Answer from the drawing. Dimensions are ordinates in mm from the lowest x, y and z of the part. A direction names the side the tool comes from. Round coordinates to 2 decimals unless told otherwise and drop trailing zeros. Loops run counter-clockwise (first coordinate to the right, second up) from the corner with the lowest first, then second, coordinate; pieces in that order, holes last. Notation, with made-up numbers: (33.25, -7.75) - (46.25, -7.75) arc R20 cw to (46.25, 16.25) - close; hole circle Ø10 at (-30.75, -10). An arc over 180 degrees is marked (long way). Use CSV: the item, a comma, the result in double quotes. Start each with the question number.
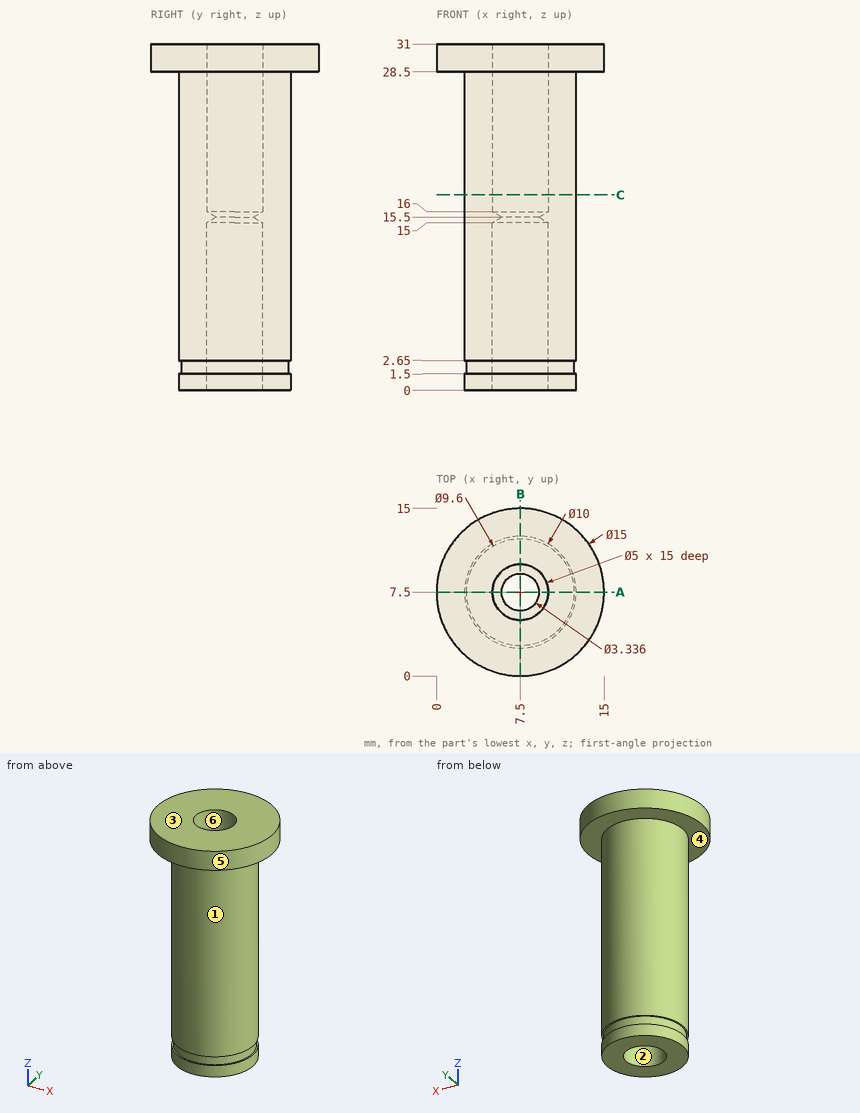
Item 1: The mould has two halves that part along Y. Classify the marked faces 1, 2 and 3: pulls with the +Y half, pulls with the -Y half, needs draft (parallel to the pull), parting line crosses it, or undercut.
Item 2: Find the intervals of material crossed by probe 1 along X at (y, z) = (7.5, 11); probe 2 along Z at (x, y) = (12, 3.25), in increasing order. Write a range as [from, to].
Item 3: Which of the six approach directions +Z, -Z, +X, -X, +Y, -Y give full straight-line access (tool end or side, diameter ignored) to the marked faces 4, 5 and 6?
Item 4: A cutting plane is placed at C-C (z = 17.5). Determine the outline of the cut face in (x, y), plus the area to 3 significant figures.
Item 5: A cutting plane is placed at A-A (y = 7.5). Determine the outline of the cut face in (x, z).
Item 6: Each of these flat-tipped pins is pushed along its axis until it touches: pin 1 Ø4 at (x, y) = (7.5, 7.5) entering from -Z; pin 2 Ø8 at (x, z) = (11.5, 22.5) entering from -Y; pin 3 Ø8 at (x, y) = (7.5, 7.5) entering from -Z; pin 4 Ø8 at (x, z) = (12, 6.5) entering from +Y (3 decimals). Where does it stop, or does it pass through?
Result sheet:
1,face 1,"parting line crosses it"
1,face 2,"undercut"
1,face 3,"needs draft"
2,probe 1,"[2.5, 5], [10, 12.5]"
2,probe 2,"[28.5, 31]"
3,face 4,"-Z"
3,face 5,"+Z, -Z"
3,face 6,"+Z"
4,outline,"circle Ø10 at (7.5, 7.5); hole circle Ø5 at (7.5, 7.5)"
4,area,"58.9 mm^2"
5,outline,"(0, 28.5) - (2.5, 28.5) - (2.5, 2.65) - (2.7, 2.65) - (2.7, 1.5) - (2.5, 1.5) - (2.5, 0) - (5, 0) - (5, 15) - (5.83, 15.5) - (5, 16) - (5, 31) - (0, 31) - close; (9.17, 15.5) - (10, 15) - (10, 0) - (12.5, 0) - (12.5, 1.5) - (12.3, 1.5) - (12.3, 2.65) - (12.5, 2.65) - (12.5, 28.5) - (15, 28.5) - (15, 31) - (10, 31) - (10, 16) - close"
6,pin 1,"z = 15.3"
6,pin 2,"y = 2.5"
6,pin 3,"z = 0"
6,pin 4,"y = 12.475"
